Source: CAD feature listing. Evaluate the final solid. Frame: model axes, mm. Coordinates: 2 decimals unless noted, no trailing zeros.
Item 1: Contact query for flat-ended pins moving along their axis: P1, Ø6.5, axis at x = -7.5, y = 1.5, coming from the +Z side; P2, Ø0.5, axis at x = 0, y = 12.5, coming from the -Z side; P3, Ø5, axis at x = -3, y = 8, coming from the +Z side. Output: stop coordinate, or through.
Item 2: Ray query, line 1 (Y direction, x = 0, z = 0.3) (3 decimals); line 2 (Y direction, x = 1, z = 0.15); line 3 (Z direction, x = -0.75, y = 5.5). Return the intervals inside material, ascending.
Item 3: Mould query, pull axis X, two halves, no side actions, for faces 1 (the flat face through (0, 0, -0.5)), 2 (the flat face through (0, 12.5, -0.3)). Classes: released by +X, released by -X, zero draft, split by the parting line, or undercut.
from build123d import *

# Parameters (mm, degrees)
SKETCH1_R           = 13
BASE_EXTRUDE_DEPTH  = 0.5
SKETCH2_R           = 4
BOSS_EXTRUDE1_DEPTH = 0.25
SKETCH3_R           = 0.09375
BOSS_EXTRUDE2_DEPTH = 0.75
SKETCH4_R           = 0.245
BOSS_EXTRUDE3_DEPTH = 1.25
SKETCH5_W           = 1
SKETCH5_H           = 2
CUT_EXTRUDE1_DEPTH  = 0.2
CHAMFER1_SIZE       = 0.1
CHAMFER2_SIZE       = 0.05
CHAMFER4_SIZE       = 0.25


with BuildPart() as part:
    # Sketch1 → Base-Extrude (new body)
    with BuildSketch(Plane.XY):
        Circle(SKETCH1_R)
    extrude(amount=-BASE_EXTRUDE_DEPTH)

    # Sketch2 → Boss-Extrude1 (add)
    with BuildSketch(Plane.XY):
        with Locations((-7.5, 0)):
            Circle(SKETCH2_R)
        with Locations((0, 7.5)):
            Circle(SKETCH2_R)
        with Locations((0, -7.5)):
            Circle(SKETCH2_R)
    extrude(amount=BOSS_EXTRUDE1_DEPTH)

    # Sketch3 → Boss-Extrude2 (add)
    with BuildSketch(Plane.XY):
        with Locations((-7.5, 0)):
            Circle(SKETCH3_R)
        with Locations((0, 7.5)):
            Circle(SKETCH3_R)
        with Locations((0, -7.5)):
            Circle(SKETCH3_R)
    extrude(amount=BOSS_EXTRUDE2_DEPTH)

    # Sketch4 → Boss-Extrude3 (add)
    with BuildSketch(Plane.XY):
        Circle(SKETCH4_R)
    extrude(amount=BOSS_EXTRUDE3_DEPTH)

    # Sketch5 → Cut-Extrude1 (cut)
    with BuildSketch(Plane(origin=(0, 0, -0.5), x_dir=(-1, 0, 0), z_dir=(0, 0, -1))):
        with Locations((0, 13)):
            Rectangle(SKETCH5_W, SKETCH5_H)
    extrude(amount=-CUT_EXTRUDE1_DEPTH, mode=Mode.SUBTRACT)

    # Chamfer1
    chamfer1_edges = [part.edges().sort_by_distance(p)[0] for p in [
        (-0.245, 0, 1.25),
    ]]
    chamfer(chamfer1_edges, length=CHAMFER1_SIZE)

    # Chamfer2
    chamfer2_edges = [part.edges().sort_by_distance(p)[0] for p in [
        (-7.59375, 0, 0.75),
        (-0.09375, 7.5, 0.75),
        (-0.09375, -7.5, 0.75),
    ]]
    chamfer(chamfer2_edges, length=CHAMFER2_SIZE)

    # Chamfer4
    chamfer4_edges = [part.edges().sort_by_distance(p)[0] for p in [
        (-13, 0, 0),
    ]]
    chamfer(chamfer4_edges, length=CHAMFER4_SIZE)


solid = part.part
Answer list:
1. P1: stops at z = 0.75
1. P2: stops at z = -0.3
1. P3: stops at z = 0.25
2. line 1: y = -7.594 to -7.406, -0.245 to 0.245, 7.406 to 7.594
2. line 2: y = -11.37 to -3.63, 3.63 to 11.37
2. line 3: z = -0.5 to 0.25
3. face 1: zero draft
3. face 2: undercut
